```python
from build123d import *

# Parameters (mm, degrees)
BOSS_EXTRUDE1_DEPTH = 6.35
CIRPATTERN1_COUNT   = 18
BOSS_EXTRUDE3_START = -6.35
BOSS_EXTRUDE3_DEPTH = 6.35
SKETCH4_R           = 1.500000048
CUT_EXTRUDE1_DEPTH  = 6.35


with BuildPart() as part:
    # Sketch1 → Boss-Extrude1 (new body)
    with BuildSketch(Plane(origin=(0, 0, 0), x_dir=(1, 0, 0), z_dir=(0, 1, 0))):
        with BuildLine():
            Line((0, 0), (-1.880045408, 10.66226734))
            ThreePointArc((-1.880045408, 10.66226734), (-1.536116928, 10.717222604), (-1.190598755, 10.761086849))
            ThreePointArc((-1.190598755, 10.761086849), (-1.022096794, 10.852519273), (-0.965497238, 11.035683923))
            Line((-0.965497238, 11.035683923), (-1.029695335, 11.769471531))
            ThreePointArc((-1.029695335, 11.769471531), (-0.972041848, 12.892396814), (-0.609362841, 13.956703655))
            ThreePointArc((-0.609362841, 13.956703655), (0, 13.97), (0.609362841, 13.956703655))
            ThreePointArc((0.609362841, 13.956703655), (0.972041848, 12.892396814), (1.029695335, 11.769471531))
            Line((1.029695335, 11.769471531), (0.965497238, 11.035683923))
            ThreePointArc((0.965497238, 11.035683923), (1.022096794, 10.852519273), (1.190598755, 10.761086849))
            ThreePointArc((1.190598755, 10.761086849), (1.536116928, 10.717222604), (1.880045408, 10.66226734))
            Line((1.880045408, 10.66226734), (0, 0))
        make_face()
    boss_extrude1 = extrude(amount=BOSS_EXTRUDE1_DEPTH)

    # CirPattern1: Boss-Extrude1 ×18 about axis
    cirpattern1_axis = Axis((0, 0, 0), (0, 1, 0))
    for i in range(1, CIRPATTERN1_COUNT):
        add(boss_extrude1.rotate(cirpattern1_axis, i * 360 / CIRPATTERN1_COUNT))

    # Sketch2 → Boss-Extrude3 (add)
    with BuildSketch(Plane(origin=(0, 6.35, 0), x_dir=(1, 0, 0), z_dir=(0, 1, 0)).offset(BOSS_EXTRUDE3_START)):
        with BuildLine():
            Line((49.084416739, -12.7), (19.05, -12.7))
            ThreePointArc((19.05, -12.7), (14.559871939, -10.840128061), (12.7, -6.35))
            Line((12.7, -6.35), (12.7, -3.175))
            Line((12.7, -3.175), (0, 0))
            Line((0, 0), (-10.559788625, -7.055555556))
            Line((-10.559788625, -7.055555556), (-1.88567654, -20.037777778))
            ThreePointArc((-1.88567654, -20.037777778), (0.400799065, -22.110173608), (3.394217772, -22.86))
            Line((3.394217772, -22.86), (82.55, -22.86))
            Line((82.55, -22.86), (82.55, -12.7))
            Line((82.55, -12.7), (74.249409051, -12.7))
            ThreePointArc((74.249409051, -12.7), (73.614409051, -12.529852263), (73.149556788, -12.065))
            Line((73.149556788, -12.065), (70.553858881, -7.569119343))
            ThreePointArc((70.553858881, -7.569119343), (61.666912895, -2.438238686), (52.77996691, -7.569119343))
            Line((52.77996691, -7.569119343), (50.184269002, -12.065))
            ThreePointArc((50.184269002, -12.065), (49.719416739, -12.529852263), (49.084416739, -12.7))
        make_face()
    extrude(amount=BOSS_EXTRUDE3_DEPTH)

    # Sketch4 → Cut-Extrude1 (cut)
    with BuildSketch(Plane(origin=(0, 6.35, 0), x_dir=(1, 0, 0), z_dir=(0, 1, 0))):
        Circle(SKETCH4_R)
    extrude(amount=-CUT_EXTRUDE1_DEPTH, mode=Mode.SUBTRACT)


solid = part.part
```
Could you check a few things on this model? Use its own coordinates, in mm. A direction names the side the tool comes from. Round coordinates to 2 decimals unless told otherwise and drop trailing zeros. Order: outer loops, then holes, each group sorted by start corner. A loop starts at its lowest first (then second) coordinate and runs counter-clockwise, first axis right, second up. Notation, with made-up numbers: M 44,74.25 L 72,74.25 A19 cw 72,90.25 Z; hole C 17.25,-8 d8. An arc over 180 degrees is marked long. One line per question, with ' | ' between items. Start each with the question number.
(1) For P1, Ø1, axis at y = 5.5, z = 1.5, coming from the +X side; P2, Ø3, axis at x = 79, y = 2, coming from the -Z side; P3, Ø3, axis at x = 8.5, y = 1, coming from the -Z side, each with a flat end and sliding along its axis, tell me the tip position at first contact or that it passes through.
(2) Suppose I cut it at B-B on z = 14. List the corners of the cut face in (x, y) for me, then the cut area to 3 significant figures.
(3) Please list where these lines run through material, in increasing order: line 1 along Z through (x, y) = (19.5, 5.75); line 2 along Z through (x, y) = (0, 4); line 3 along X through (y, z) = (3, 5.5).
(4) Thinking about a two-plate mould opening in Z: for faces 5 (the face through (61.82, 3.13, 2.44)), 6 (the face through (-12.512, 3.131, 3.196)), 7 (the face through (23, 0, 16)), which applies, +Z half, -Z half, draft (parallel to the pull), parting line (faces both ways), or undercut?
(5) Suppose I cut it at A-A on x = 24.5. List the corners of the cut face in (y, z) for me, then the cut area to 3 significant figures.
(6) For faces 1 (the face through (-9.024, 3.131, -9.238)), 2 (the face through (34, 3, 12.7)), 3 (the face through (11.66, 3.13, -5.61)), 4 (the face through (-5.32, 3.13, -11.77)), which set-ups out of +Z, -Z, +X, -X, +Y, -Y let a thin tool reach every point of the face, with its end or its side?
Geometry results:
1) P1: x = 13.85 | P2: z = 12.7 | P3: z = -11.08
2) outline: M -5.92,0 L 82.55,0 L 82.55,6.35 L -5.92,6.35 Z | area: 562 mm²
3) line 1: 12.7 to 22.86 | line 2: -13.97 to -1.5, 1.5 to 21.88 | line 3: -11.53 to 12.7, 54.36 to 68.98
4) face 5: -Z half | face 6: undercut | face 7: draft
5) outline: M 0,12.7 L 6.35,12.7 L 6.35,22.86 L 0,22.86 Z | area: 64.5 mm²
6) face 1: -X, +Y, -Y | face 2: -Z, +Y, -Y | face 3: +X, +Y, -Y | face 4: +Y, -Y
